```python
from build123d import *

# Parameters (mm, degrees)
SKETCH1_R           = 10.25
BOSS_EXTRUDE1_DEPTH = 2
SKETCH2_R           = 4.4
SKETCH2_R_2         = 2.9
BOSS_EXTRUDE2_DEPTH = 3.5
FILLET1_SIZE        = 1
FILLET1_SIZE_2      = 3
SKETCH3_R           = 1.5
CUT_EXTRUDE1_DEPTH  = 2


with BuildPart() as part:
    # Sketch1 → Boss-Extrude1 (new body)
    with BuildSketch(Plane(origin=(0, 0, 0), x_dir=(1, 0, 0), z_dir=(0, 1, 0))):
        with Locations(Location((0, 0, 0), (0, 0, 270))):
            Circle(SKETCH1_R)
    extrude(amount=BOSS_EXTRUDE1_DEPTH)

    # Sketch2 → Boss-Extrude2 (add)
    with BuildSketch(Plane(origin=(0, 2, 0), x_dir=(1, 0, 0), z_dir=(0, 1, 0))):
        with Locations(Location((0, 0, 0), (0, 0, 270))):
            Circle(SKETCH2_R)
        with Locations(Location((0, 0, 0), (0, 0, 270))):
            Circle(SKETCH2_R_2, mode=Mode.SUBTRACT)
    extrude(amount=BOSS_EXTRUDE2_DEPTH)

    # Fillet1
    # an asymmetric fillet: 3, 1 mm, written as the material it adds along each edge
    with BuildSketch(Plane(origin=(0, 2, 0), x_dir=(0, 0, 1), z_dir=(-1, 0, 0))) as fillet1_piece_1:
        with BuildLine():
            Bezier((4.4 + FILLET1_SIZE, 0), (4.4, 0), (4.4, FILLET1_SIZE_2), weights=[1, 0.707106781, 1])
            Line((4.4, FILLET1_SIZE_2), (4.4, 0))
            Line((4.4, 0), (4.4 + FILLET1_SIZE, 0))
        make_face()
    revolve(axis=Axis((0, 2, 0), (0, 1, 0)))

    # Sketch3 → Cut-Extrude1 (cut)
    with BuildSketch(Plane.XZ):
        with Locations(Location((0, 0, 0), (0, 0, 270))):
            Circle(SKETCH3_R)
    extrude(amount=-CUT_EXTRUDE1_DEPTH, mode=Mode.SUBTRACT)


solid = part.part
```
Read the model definition and answer for the solid it produces. Units are mm, in the model's axes. A direction names the side the tool comes from. Round coordinates to 2 decimals unless told otherwise and drop trailing zeros. Write each loop counter-clockwise with the first axis right and the second up, starting at its lowest first coordinate (ties: lowest second). Pieces come first, ordered by that corner, then holes. Notation, with made-up numbers: (9.25, 52) - (54.25, 52) arc R26 ccw to (54.25, 90) - close; hole circle Ø1 at (4, 39). An arc over 180 degrees is marked (long way). One line per item, written item: value.
Q1. Find section C-C (x = 9.25). Determine the outline of the cut face in (y, z).
The answers:
outline: (0, -4.42) - (2, -4.42) - (2, 4.42) - (0, 4.42) - close
Q2. Which of the six approach directions +Z, -Z, +X, -X, +Y, -Y give full straight-line access (tool end or side, diameter ignored) to faces 4 (the flat face through (-1.2, 2, 1.2)), 5 (the flat face through (-3, 5.5, 1))?
The answers:
face 4: +Y
face 5: +Z, -Z, +X, -X, +Y
Q3. This flat-tipped pin is pushed along its axis until it touches: P1, Ø1.5, axis at x = -1.5, z = 0, coming from the +Y side. Where does it stop, or does it pass through?
The answers:
P1: stops at y = 2
Q4. Find section A-A (y = 1.6). Determine the outline of the cut face in (x, z).
The answers:
outline: circle Ø20.5 at (0, 0); hole circle Ø3 at (0, 0)
Q5. For a pull along Z with two mould halves and no side action, classify faces 1 (the cylindrical face through (0.1, 3.7, -2.9)), 2 (the flat face through (-4, 2, 4)), 3 (the cylindrical face through (-10.006, 0.986, -2.222)) as pulls with the +Z half, pulls with the -Z half, needs draft (parallel to the pull), parting line crosses it, or undercut.
The answers:
face 1: undercut
face 2: needs draft
face 3: parting line crosses it
Q6. Find section B-B (x = 6.5). Determine the outline of the cut face in (y, z), and give its area (3 significant figures).
The answers:
outline: (0, -7.93) - (2, -7.93) - (2, 7.93) - (0, 7.93) - close
area: 31.7 mm2
Q7. Straight lines are drawn through the part: line 1 (Y direction, x = 8.5, z = -0.25); line 2 (Z direction, x = 2.5, y = 4.2); line 3 (Z direction, x = -1.5, y = 5.1). For each, find the intervals that lie inside material, in ascending order. Write a range as from..to.
The answers:
line 1: y = 0..2
line 2: z = -3.66..-1.47, 1.47..3.66
line 3: z = -4.14..-2.48, 2.48..4.14
